from build123d import *

# Parameters (mm, degrees)
SKETCH1_W           = 1676.4
SKETCH1_H           = 133.35
BOSS_EXTRUDE1_DEPTH = 133.35
SKETCH2_W           = 107.95
SKETCH2_H           = 107.95
CUT_EXTRUDE1_DEPTH  = 1524
SKETCH3_W           = 107.95
SKETCH3_H           = 107.95
BOSS_EXTRUDE2_DEPTH = 114.3
SKETCH4_W           = 114.3
SKETCH4_H           = 342.9
BOSS_EXTRUDE3_DEPTH = 12.7
SKETCH5_W           = 114.3
SKETCH5_H           = 12.7
BOSS_EXTRUDE4_DEPTH = 101.6
SKETCH6_R           = 31.75
BOSS_EXTRUDE5_DEPTH = 317.5
SKETCH7_R           = 6.35
CUT_EXTRUDE2_DEPTH  = 12.7


with BuildPart() as part:
    # Sketch1 → Boss-Extrude1 (new body)
    with BuildSketch(Plane.XY):
        with Locations((838.2, 66.675)):
            Rectangle(SKETCH1_W, SKETCH1_H)
    extrude(amount=BOSS_EXTRUDE1_DEPTH)

    # Sketch2 → Cut-Extrude1 (cut)
    with BuildSketch(Plane(origin=(1676.4, 0, 0), x_dir=(0, 0, -1), z_dir=(1, 0, 0))):
        with Locations((-66.675, 66.675)):
            Rectangle(SKETCH2_W, SKETCH2_H)
    extrude(amount=-CUT_EXTRUDE1_DEPTH, mode=Mode.SUBTRACT)

    # Sketch3 → Boss-Extrude2 (add)
    with BuildSketch(Plane(origin=(0, 133.35, 0), x_dir=(1, 0, 0), z_dir=(0, 1, 0))):
        with Locations((79.375, -66.675)):
            Rectangle(SKETCH3_W, SKETCH3_H)
    extrude(amount=BOSS_EXTRUDE2_DEPTH)

    # Sketch4 → Boss-Extrude3 (add)
    with BuildSketch(Plane(origin=(0, 247.65, 0), x_dir=(1, 0, 0), z_dir=(0, 1, 0))):
        with Locations((82.55, -69.85)):
            Rectangle(SKETCH4_W, SKETCH4_H)
    extrude(amount=BOSS_EXTRUDE3_DEPTH)

    # Sketch5 → Boss-Extrude4 (add)
    with BuildSketch(Plane(origin=(0, 260.35, 0), x_dir=(1, 0, 0), z_dir=(0, 1, 0))):
        with Locations((82.55, 95.25)):
            Rectangle(SKETCH5_W, SKETCH5_H)
        with Locations((82.55, -234.95)):
            Rectangle(SKETCH5_W, SKETCH5_H)
    extrude(amount=BOSS_EXTRUDE4_DEPTH)

    # Sketch6 → Boss-Extrude5 (add)
    with BuildSketch(Plane.XY.offset(-88.9)):
        with Locations((82.55, 304.8)):
            Circle(SKETCH6_R)
    extrude(amount=BOSS_EXTRUDE5_DEPTH)

    # Sketch7 → Cut-Extrude2 (cut)
    with BuildSketch(Plane(origin=(0, 133.35, 0), x_dir=(1, 0, 0), z_dir=(0, 1, 0))):
        with Locations((196.85, -66.675)):
            Circle(SKETCH7_R)
        with Locations((1638.3, -66.675)):
            Circle(SKETCH7_R)
    extrude(amount=-CUT_EXTRUDE2_DEPTH, mode=Mode.SUBTRACT)


solid = part.part
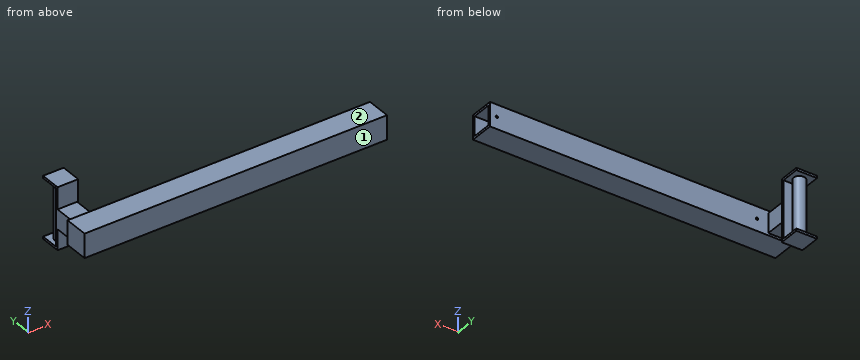
For this review, take the finished solid that the model builds, in its own axes (mm). Face numbers are marked on the shaded views. Coordinates: 2 decimals unless noted, no trailing zeros. Order: outer loops, then holes, each group sorted by start corner. A loop starts at its lowest first (then second) coordinate and runs counter-clockwise, first axis right, second up. Notation, with made-up numbers: (13, 1) -> (53, 1) arc R26 ccw to (53, 36) -> close; hole circle Ø4 at (1, 77.25). An arc over 180 degrees is marked (long way). Return JSON: item names as keys, results as strings.
1. For pin 1 Ø8 at (x, y) = (721, 99) entering from -Z, flat-tipped, find the tip position at first contact; note if it passes through.
Answer block:
{"pin 1": "z = 0"}
2. For line 1 (Z direction, x = 1175, y = 48); line 2 (Z direction, x = 196.85, y = 127.25) (3 decimals), list the stretches that pass through material, from the lowest coordinate up. Write a range as from..to.
Answer block:
{"line 1": "0..12.7, 120.65..133.35", "line 2": "0..60.325, 73.025..133.35"}
3. We need section B-B on z = -36.5. Write out the cut boundary in (x, y), and give its area (3 significant figures).
Answer block:
{"outline": "(25.4, 247.65) -> (139.7, 247.65) -> (139.7, 260.35) -> (25.4, 260.35) -> close; circle Ø63.5 at (82.55, 304.8)", "area": "4,620 mm²"}
4. We need section D-D on x = 82.55. Write out the cut boundary in (y, z), and give its area (3 significant figures).
Answer block:
{"outline": "(0, 0) -> (133.35, 0) -> (133.35, 12.7) -> (247.65, 12.7) -> (247.65, -101.6) -> (361.95, -101.6) -> (361.95, -88.9) -> (336.55, -88.9) -> (336.55, 228.6) -> (361.95, 228.6) -> (361.95, 241.3) -> (247.65, 241.3) -> (247.65, 120.65) -> (133.35, 120.65) -> (133.35, 133.35) -> (0, 133.35) -> close; hole (260.35, -88.9) -> (273.05, -88.9) -> (273.05, 228.6) -> (260.35, 228.6) -> close", "area": "57,200 mm²"}
5. We need section C-C on y = 304.8. Write out the cut boundary in (x, z), and give its area (3 significant figures).
Answer block:
{"outline": "(25.4, -101.6) -> (139.7, -101.6) -> (139.7, -88.9) -> (114.3, -88.9) -> (114.3, 228.6) -> (139.7, 228.6) -> (139.7, 241.3) -> (25.4, 241.3) -> (25.4, 228.6) -> (50.8, 228.6) -> (50.8, -88.9) -> (25.4, -88.9) -> close", "area": "23,100 mm²"}
6. We need section A-A on x = 615. Write out the cut boundary in (y, z), and give its area (3 significant figures).
Answer block:
{"outline": "(0, 0) -> (133.35, 0) -> (133.35, 133.35) -> (0, 133.35) -> close; hole (12.7, 12.7) -> (120.65, 12.7) -> (120.65, 120.65) -> (12.7, 120.65) -> close", "area": "6,130 mm²"}
7. The part is to be moulded in two halves that separate along Y. For the marked faces 1 and 2, say which applies: +Y half, -Y half, draft (parallel to the pull), parting line (faces both ways), or undercut.
Answer block:
{"face 1": "-Y half", "face 2": "draft"}
